Verification items for the finished model (mm, model axes). Round coordinates to 2 decimals unless told otherwise and drop trailing zeros. Write each loop counter-clockwise with the first axis right and the second up, starting at its lowest first coordinate (ties: lowest second). Pieces come first, ordered by that corner, then holes. Notation, with made-up numbers: M -23.75,59 L -14.75,59 A16 cw -14.75,70 Z; hole C -8.5,79 d10. An arc over 180 degrees is marked long. One line per item, written item: value. Start each with the question number.
Item 1: Section check A-A, the plane z = 51.5. Record the cut outline in (x, y), then the cut area to 3 significant figures.
Item 2: Thickness scan on probe 1 along Y at (x, z) = (0.5, 255); probe 2 along X at (y, z) = (1.7, 127); probe 3 along X at (y, z) = (2.2, 141). Record the ranges inside material, lowest first. Write a range as from..to.
Item 3: Gauge pin test, flat ends, axial feed: pin 1 (0.7 mm diameter, centred on x = 4, z = 148.5, fed in from -Y); pin 2 (0.7 mm diameter, centred on x = -4.5, z = 237, fed in from -Y); pin 3 (1.5 mm diameter, centred on x = -0.5, y = 1.5, fed in from +Z). Record the tip position at first contact, or that the pin passes through.
from build123d import *

# Parameters (mm, degrees)
PAD_DEPTH = 340


with BuildPart() as part:
    # Sketch → Pad (new body)
    with BuildSketch(Plane.XY):
        with BuildLine():
            Line((-4.5, 4.3), (4.5, 4.3))
            Line((4.5, 4.3), (4.5, 4))
            Line((4.5, 4), (3.9, 4))
            Line((3.9, 4), (4.5, 2))
            Line((4.5, 2), (3.441966, 0))
            ThreePointArc((2.558034, 0.467615), (2.766192, -0.208159), (3.441966, 0))
            Line((2.558034, 0.467615), (3.368691, 2))
            Line((3.368691, 2), (3, 3.228972))
            Line((-3, 3.228972), (3, 3.228972))
            Line((-3, 3.228972), (-3.368691, 2))
            Line((-3.368691, 2), (-2.558034, 0.467615))
            ThreePointArc((-3.441966, 0), (-2.766192, -0.208159), (-2.558034, 0.467615))
            Line((-3.441966, 0), (-4.5, 2))
            Line((-4.5, 2), (-3.9, 4))
            Line((-3.9, 4), (-4.5, 4))
            Line((-4.5, 4), (-4.5, 4.3))
        make_face()
    extrude(amount=PAD_DEPTH)


solid = part.part
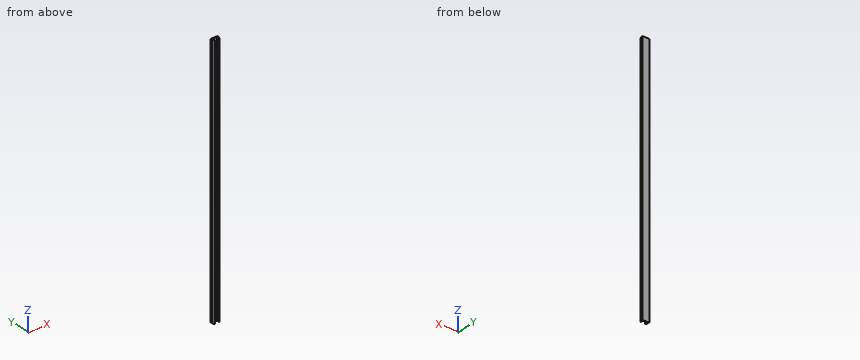
Response values:
1. outline: M -4.5,2 L -3.44,0 A0.5 ccw -2.56,0.47 L -3.37,2 L -3,3.23 L 3,3.23 L 3.37,2 L 2.56,0.47 A0.5 ccw 3.44,0 L 4.5,2 L 3.9,4 L 4.5,4 L 4.5,4.3 L -4.5,4.3 L -4.5,4 L -3.9,4 Z
1. area: 16.5 mm2
2. probe 1: y = 3.23..4.3
2. probe 2: x = -4.34..-3.21, 3.21..4.34
2. probe 3: x = -4.44..-3.31, 3.31..4.44
3. pin 1: stops at y = 0.39
3. pin 2: stops at y = 1.34
3. pin 3: passes through
